Could you check a few things on this model? Use its own coordinates, in mm. Face numbers are marked on the shaded views. A direction names the side the tool comes from. Round coordinates to 2 decimals unless told otherwise and drop trailing zeros. Order: outer loops, then holes, each group sorted by start corner. A loop starts at its lowest first (then second) coordinate and runs counter-clockwise, first axis right, second up. Notation, with made-up numbers: (15, 25) -> (53, 25) arc R18 ccw to (53, 56) -> close; hole circle Ø1 at (64, 77.25). An arc over 180 degrees is marked (long way). One line per question, with ' | ' between items.
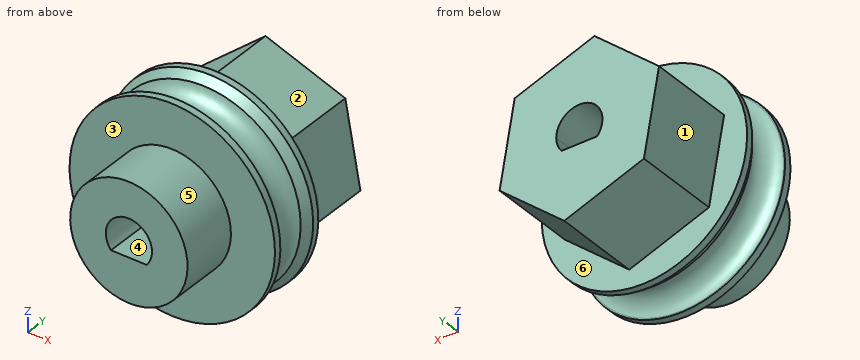
```python
from build123d import *

# Parameters (mm, degrees)
BOSS_EXTRUDE1_DEPTH    = 7.62
MOTOR_SHAFT_DEPTH      = 17.164461018
MOTOR_SHAFT_DEPTH_BACK = 17.164461018


with BuildPart() as part:
    # Sketch1 → Boss-Extrude1 (new body)
    with BuildSketch(Plane(origin=(0, 0, 0), x_dir=(1, 0, 0), z_dir=(0, 1, 0))):
        Polygon((6.902283212, 2.474231151), (1.308394574, 7.214668182), (-5.593888638, 4.74043703), (-6.902283212, -2.474231151), (-1.308394574, -7.214668182), (5.593888638, -4.74043703), align=None)
    extrude(amount=BOSS_EXTRUDE1_DEPTH)

    # Sketch5 → Revolve1 (revolve)
    with BuildSketch(Plane(origin=(0, 0, 0), x_dir=(0, 0, -1), z_dir=(1, 0, 0)), mode=Mode.PRIVATE) as revolve1_sk:
        with BuildLine():
            Line((0, 0), (-8.89, 0))
            Line((-8.89, 0), (-8.89, -1.27))
            Line((-8.89, -1.27), (-8.763, -1.27))
            ThreePointArc((-8.763, -1.27), (-7.1755, -2.8575), (-8.763, -4.445))
            Line((-8.763, -4.445), (-8.89, -4.445))
            Line((-8.89, -4.445), (-8.89, -5.08))
            Line((-8.89, -5.08), (-5.08, -5.08))
            Line((-5.08, -5.08), (-5.08, -10.16))
            Line((-5.08, -10.16), (0, -10.16))
            Line((0, -10.16), (0, -5.08))
            Line((0, -5.08), (0, 0))
        make_face()
    revolve(revolve1_sk.sketch.rotate(Axis((0, 0, 0), (0, 1, 0)), 180), axis=Axis((0, 0, 0), (0, 1, 0)))

    # Chamfer5: read off the stored shape, not the designer's step
    # Chamfer5 outline → Chamfer5 (revolve, cut)
    with BuildSketch(Plane.XY):
        Polygon((8.339893048, -1.32742263), (8.763, -1.32742263), (8.763, -1.27), (8.89, -1.27), (8.89, -0.604551432), align=None)
    revolve(axis=Axis((0, 0, 0), (0, 1, 0)), mode=Mode.SUBTRACT)

    # Sketch10 → motor shaft (cut, two sides: drawn at the far end of the back side and taken through both)
    with BuildSketch(Plane(origin=(0, 0, 0), x_dir=(1, 0, 0), z_dir=(0, 1, 0)).offset(-MOTOR_SHAFT_DEPTH_BACK)):
        with BuildLine():
            Line((1.545024355, 1.27), (-1.545024355, 1.27))
            ThreePointArc((-1.545024355, 1.27), (-0.674518883, -1.882823553), (2.000000064, 0))
            ThreePointArc((2.000000064, 0), (1.882823553, 0.674518883), (1.545024355, 1.27))
        make_face()
    extrude(amount=MOTOR_SHAFT_DEPTH + MOTOR_SHAFT_DEPTH_BACK, mode=Mode.SUBTRACT)


solid = part.part
```
1. I'm going to push flat-ended pins straight in: pin 1 (1 mm diameter, centred on y = 0, z = -3.5, fed in from +X); pin 2 (1.5 mm diameter, centred on x = -4.5, y = -6, fed in from -Z); pin 3 (3 mm diameter, centred on x = 6.5, y = -0.5, fed in from -Z). Where does each tip first touch, or does it pass through?
From the geometry:
pin 1: stops at x = 8.37 | pin 2: stops at z = -3.43 | pin 3: stops at z = -7.35
2. I want a section at C-C on y = -4. List the corners of the cut face in (x, z) for me.
From the geometry:
outline: circle Ø15.32 at (0, 0); hole (-1.55, -1.27) -> (1.55, -1.27) arc R2 ccw (long way) to start
3. If we mould it in two halves opening along X, with no side actions, what happens to the marked faces 4, 5 and 6? For each: pulls with the +X half, pulls with the -X half, needs draft (parallel to the pull), parting line crosses it, or undercut.
From the geometry:
face 4: undercut | face 5: parting line crosses it | face 6: needs draft
4. I want a section at A-A on y = 2.75. List the corners of the cut face in (x, z) for me, and give its area (3 significant figures).
From the geometry:
outline: (-6.9, 2.47) -> (-5.59, -4.74) -> (1.31, -7.21) -> (6.9, -2.47) -> (5.59, 4.74) -> (-1.31, 7.21) -> close; hole (-1.55, -1.27) -> (1.55, -1.27) arc R2 ccw (long way) to start | area: 129 mm²
5. On a 3-axis mill with a long thin cutter (end or side, diameter ignored), from which of +Z, -Z, +X, -X, +Y, -Y can I reach the whole of each face in a straight line? I mean the marked faces 1, 2 and 3. Say none if no direction works.
From the geometry:
face 1: -Z, -X, +Y | face 2: +Z, +X, +Y | face 3: -Y
6. I need wall thicknesses on probe 1 along Z at (x, y) = (0, -0.5); probe 2 along Y at (x, z) = (0.5, 5.5); probe 3 along Y at (x, z) = (-5.75, 3.5). Which ranges of each line are inside material? Lowest first, please.
From the geometry:
probe 1: z = -8.89 to -1.27, 2 to 8.89 | probe 2: y = -5.08 to 7.62 | probe 3: y = -5.08 to 0
